Autodesk Fusion 360 part; units mm, degrees
sketch "草图1" plane through (0, 0, 0) normal (0, 0, 1) x (1, 0, 0)
  arc A0 (-2.4024, -17.839) -> (2.4024, -17.839) centre (0, 0) ccw
  line L0 (0, 0) -> (0, -48) construction
  line L1 (14.2478, 11) -> (-14.2478, 11)
  line L2 (2.4024, -17.839) -> (16.6502, 6.839)
  arc A1 (-14.2478, 11) -> (-16.6502, 6.839) centre (0, 0) ccw
  line L3 (-16.6502, 6.839) -> (-2.4024, -17.839)
  arc A2 (16.6502, 6.839) -> (14.2478, 11) centre (0, 0) ccw
  circle A3 centre (0, 0) radius 43
extrude "拉伸1" add sketch "草图1" against normal blind 2 contours A0 L1 L2 A1 L3 A2 | A3 makes body 1
extrude "拉伸2" add sketch "草图1" along normal blind 8 contours A0 L1 L2 A1 L3 A2 bodies 1
copy_body "实体->零部件1" bodies 1 removing the originals makes body 2 in component "Component'"
sketch "草图2" plane through (0, 0, -2) normal (0, 0, -1) x (1, 0, 0)
  circle A0 centre (0, 0) radius 43
  circle A1 centre (0, 0) radius 29.5
  circle A2 centre (0, 0) radius 24
  dimension "d11" = 59
  dimension "d12" = 48
extrude "拉伸1'" cut sketch "草图2" against normal blind 1 contours A1 bodies 2 in component "Component'"
component "Component'" placed x (1, 0, 0) y (0, 1, 0) z (0, 0, 1) at (0, 0, 0)
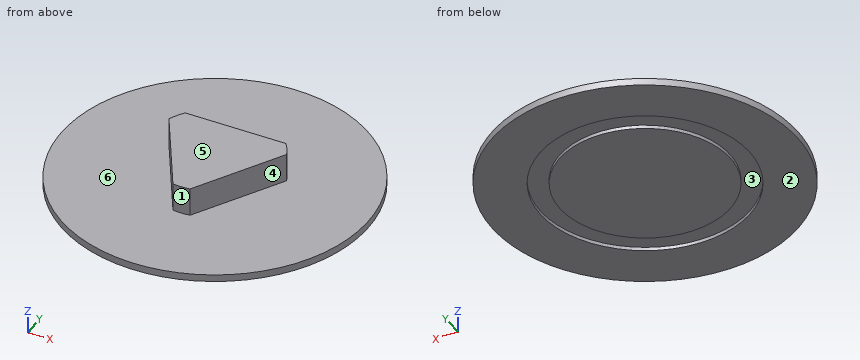
Design review of the part built by this model. Coordinates are the model's own, in mm. Face numbers are marked on the shaded views. A direction names the side the tool comes from. Coordinates: 2 decimals unless noted, no trailing zeros. Write each loop counter-clockwise with the first axis right and the second up, starting at its lowest first coordinate (ties: lowest second). Pieces come first, ordered by that corner, then holes.
1) Mouldability with a two-part tool opening along X and no side actions: class the marked faces 1, 2 and 3 as +X half, -X half, draft (parallel to the pull), parting line (faces both ways), or undercut.
2) Machinability: for the marked faces 4, 5 and 6, which of the approach directions +Z, -Z, +X, -X, +Y, -Y give a long, thin tool a straight path to every point of the face, cutting with its end or side? Answer none if there is none.
3) To check wall thickness, follow L1, parallel to Y at x = 0, z = -1.5; L2, parallel to Z at x = 37.5, y = 14.5; L3, parallel to Z at x = -27, y = 8. State the ranges of each line that lie inside material, in increasing order.
4) Add section B-B (x = 6). Write out the cut boundary in (y, z).
5) Add section D-D (x = -35). Write out the cut boundary in (y, z).
6) Add section A-A (z = 2.25). Write out the cut boundary in (x, y).
7) Insertion check: pin 1 (5 mm diameter, centred on x = 10, z = 1, fed in from +Y); pin 2 (8 mm diameter, centred on x = 19.5, y = -18.5, fed in from +Z); pin 3 (3 mm diameter, centred on x = 15.5, z = 5, fed in from +Y); pin 4 (6 mm diameter, centred on y = 16.5, z = 6, fed in from -X). Each pin has a flat end and moves straight along its axis. Give the tip position at first contact, or say it passes through.
8) Add section C-C (y = 0). Write out the cut boundary in (x, z).
Check result:
1. face 1: parting line
1. face 2: draft
1. face 3: undercut
2. face 4: +Z, +X, -Y
2. face 5: +Z, +X, -X, +Y, -Y
2. face 6: +Z
3. L1: y = -43 to -29.5, -24 to 24, 29.5 to 43
3. L2: z = -2 to 0
3. L3: z = -1 to 0
4. outline: (-42.58, -2) - (-28.88, -2) - (-28.88, -1) - (-23.24, -1) - (-23.24, -2) - (23.24, -2) - (23.24, -1) - (28.88, -1) - (28.88, -2) - (42.58, -2) - (42.58, 0) - (11, 0) - (11, 8) - (-11.61, 8) - (-11.61, 0) - (-42.58, 0) - close
5. outline: (-24.98, -2) - (24.98, -2) - (24.98, 0) - (-24.98, 0) - close
6. outline: (-16.65, 6.84) - (-2.4, -17.84) arc R18 ccw to (2.4, -17.84) - (16.65, 6.84) arc R18 ccw to (14.25, 11) - (-14.25, 11) arc R18 ccw to start
7. pin 1: stops at y = 42.3
7. pin 2: stops at z = 0
7. pin 3: stops at y = 11
7. pin 4: passes through
8. outline: (-43, -2) - (-29.5, -2) - (-29.5, -1) - (-24, -1) - (-24, -2) - (24, -2) - (24, -1) - (29.5, -1) - (29.5, -2) - (43, -2) - (43, 0) - (12.7, 0) - (12.7, 8) - (-12.7, 8) - (-12.7, 0) - (-43, 0) - close
